```python
from build123d import *

# Parameters (mm, degrees)
F0_R     = 31.75
F1_DEPTH = 5.95376
F2_R     = 14.39799
F3_DEPTH = 13.09624
F5_R     = 2.38125
F6_DEPTH = 5.95476
F4_R     = 11.9126
F7_DEPTH = 15.24


with BuildPart() as f1:
    # F0 (on Top) → F1 (new body)
    with BuildSketch(Plane.XY):
        Circle(F0_R)
    extrude(amount=-F1_DEPTH)

    # F2 (on face) → F3 (join)
    with BuildSketch(Plane.XY):
        Circle(F2_R)
    extrude(amount=F3_DEPTH)

    # F5 (on face) → F6 (cut, through all)
    with BuildSketch(Plane.XY):
        with Locations((-23.8252, 0)):
            Circle(F5_R)
        with Locations((-11.9126, 20.633228)):
            Circle(F5_R)
        with Locations((11.9126, 20.633228)):
            Circle(F5_R)
        with Locations((23.8252, 0)):
            Circle(F5_R)
        with Locations((11.9126, -20.633228)):
            Circle(F5_R)
        with Locations((-11.9126, -20.633228)):
            Circle(F5_R)
    extrude(amount=-F6_DEPTH, mode=Mode.SUBTRACT)

    # F4 (on face) → F7 (cut)
    with BuildSketch(Plane.XY.offset(13.09624)):
        Circle(F4_R)
    extrude(amount=-F7_DEPTH, mode=Mode.SUBTRACT)


solid = f1.part
```
Build history of the part. All positions in model axes, mm. A direction names the side the tool comes from. Give positions to 0.01 mm unless a question says otherwise; leave off trailing zeros. Order: outer loops, then holes, each group sorted by start corner. A loop starts at its lowest first (then second) coordinate and runs counter-clockwise, first axis right, second up. Notation, with made-up numbers: M -38,72.5 L 17,72.5 A17 ccw 17,92.5 Z; hole C 49.25,35 d5. An arc over 180 degrees is marked long. Write item = value, one per line. Start each with the question number.
(1) Pin check, flat tips, straight feed: pin 1 Ø6 at (x, y) = (11.91, -20.63) entering from +Z; pin 2 Ø4 at (x, z) = (-10.5, 8.5) entering from -Y; pin 3 Ø1.5 at (y, z) = (7, 7.5) entering from -X. Stop position of each tip, or through.
(2) Which spindle directions (+Z, -Z, +X, -X, +Y, -Y) get a long thin tool onto all of the face, cutting with end or side? Do faces 1 (the cylindrical face through (-21.554, 0.715, -2.935)), 2 (the cylindrical face through (-9.45, -7.25, 5.58)). Say none if no direction does.
(3) Probe L1, parallel to Z at x = 7.5, y = -5; L2, parallel to X at y = 7, z = 7.5; L3, parallel to X at y = -8.5, z = 6.75. List the from-to ranges inside material, lowest first. Write a range as [from, to].
(4) Two-plate mould, pull along Y, no slides. Class faces 3 (the cylindrical face through (-6.883, -30.995, -2.935)), 4 (the cylindrical face through (26.1, 0.7, -2.9)), 5 (the flat face through (0, 0, -5.954)): released by +Y, released by -Y, zero draft, split by the parting line, or undercut.
(5) Slice it at A-A on y = 0. Write the cut outline in (x, z), plus the area to 3 significant figures.
(6) Slice it at C-C on z = 10.75. Write the cut outline in (x, y).
(7) Slice it at D-D on x = 0. Write the cut outline in (y, z), plus the area to 3 significant figures.
(8) Slice it at B-B on x = 25. Write the cut outline in (y, z), plus the area to 3 significant figures.
Responses:
q1.pin_1 = 0
q1.pin_2 = -11.62
q1.pin_3 = -12.97
q2.face_1 = +Z, -Z
q2.face_2 = +Z
q3.L1 = [-5.95, -2.14]
q3.L2 = [-12.58, -9.64], [9.64, 12.58]
q3.L3 = [-11.62, -8.35], [8.35, 11.62]
q4.face_3 = split by the parting line
q4.face_4 = undercut
q4.face_5 = zero draft
q5.outline = M -31.75,-5.95 L -26.21,-5.95 L -26.21,0 L -31.75,0 Z; M -21.44,-5.95 L 21.44,-5.95 L 21.44,0 L 14.4,0 L 14.4,13.1 L 11.91,13.1 L 11.91,-2.14 L -11.91,-2.14 L -11.91,13.1 L -14.4,13.1 L -14.4,0 L -21.44,0 Z; M 26.21,-5.95 L 31.75,-5.95 L 31.75,0 L 26.21,0 Z
q5.area = 335 mm2
q6.outline = C 0,0 d28.8; hole C 0,0 d23.83
q7.outline = M -31.75,-5.95 L 31.75,-5.95 L 31.75,0 L 14.4,0 L 14.4,13.1 L 11.91,13.1 L 11.91,-2.14 L -11.91,-2.14 L -11.91,13.1 L -14.4,13.1 L -14.4,0 L -31.75,0 Z
q7.area = 392 mm2
q8.outline = M -19.57,-5.95 L -2.07,-5.95 L -2.07,0 L -19.57,0 Z; M 2.07,-5.95 L 19.57,-5.95 L 19.57,0 L 2.07,0 Z
q8.area = 208 mm2
